Build history of the part. All positions in model axes, mm. Face numbers are marked on the shaded views. A direction names the side the tool comes from. Give positions to 0.01 mm unless a question says otherwise; leave off trailing zeros. Order: outer loops, then holes, each group sorted by start corner. A loop starts at its lowest first (then second) coordinate and runs counter-clockwise, first axis right, second up. Notation, with made-up numbers: M 81.25,16 L 85.25,16 A27 ccw 85.25,45 Z; hole C 53.5,59 d7. An arc over 180 degrees is marked long. One line per item, written item: value.
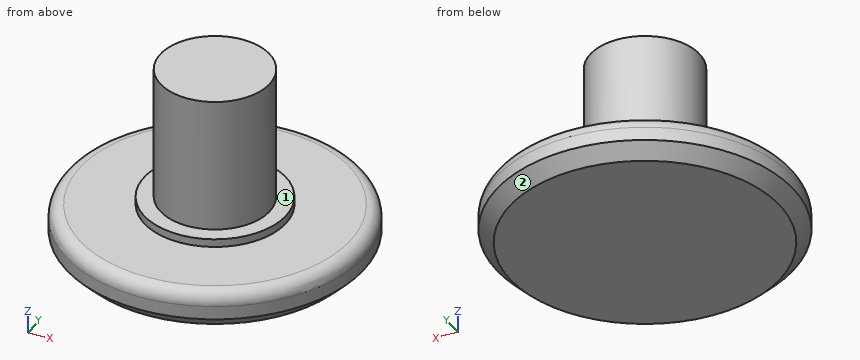
from build123d import *

# Parameters (mm, degrees)
F0_R     = 11
F1_DEPTH = 3
F2_R     = 5.25
F3_DEPTH = 0.6
F4_R     = 4.05
F5_DEPTH = 10
F6_SIZE  = 1
F7_R     = 1


with BuildPart() as f1:
    # F0 (on Top) → F1 (new body)
    with BuildSketch(Plane.XY):
        Circle(F0_R)
    extrude(amount=F1_DEPTH)

    # F2 (on face) → F3 (join)
    with BuildSketch(Plane.XY.offset(3)):
        Circle(F2_R)
    extrude(amount=F3_DEPTH)

    # F4 (on face) → F5 (join)
    with BuildSketch(Plane.XY.offset(3.6)):
        Circle(F4_R)
    extrude(amount=F5_DEPTH)

    # F6
    f6_edges = [f1.edges().sort_by_distance(p)[0] for p in [
        (-11, 0, 0),
    ]]
    chamfer(f6_edges, length=F6_SIZE)

    # F7
    f7_edges = [f1.edges().sort_by_distance(p)[0] for p in [
        (-11, 0, 3),
    ]]
    fillet(f7_edges, radius=F7_R)


solid = f1.part
1) Saw through at A-A, the plane y = 0. Write the cut outline in (x, z).
Check values:
outline: M -11,1 L -10,0 L 10,0 L 11,1 L 11,2 A1 ccw 10,3 L 5.25,3 L 5.25,3.6 L 4.05,3.6 L 4.05,13.6 L -4.05,13.6 L -4.05,3.6 L -5.25,3.6 L -5.25,3 L -10,3 A1 ccw -11,2 Z
2) Tool access for the marked faces 1 and 2: list every direction of +Z, -Z, +X, -X, +Y, -Y with a clear straight run to the whole face (end or side of a thin tool).
Check values:
face 1: +Z
face 2: -Z
3) Pin check, flat tips, straight feed: pin 1 (1.5 mm diameter, centred on x = 4.5, z = 2.5, fed in from -Y); pin 2 (4 mm diameter, centred on y = -6, z = 3, fed in from +X); pin 3 (3 mm diameter, centred on x = -1.5, z = 5, fed in from +Y). Stop position of each tip, or through.
Check values:
pin 1: y = -10.3
pin 2: x = 10.16
pin 3: y = 5.16
4) Drill centre lines: probe 1 along Z at (x, y) = (1.5, -4); probe 2 along Z at (x, y) = (-3.25, 7); probe 3 along Y at (x, z) = (2.5, 9.5). Where is each one in solid material? Low to high. Write a range as from..to.
Check values:
probe 1: 0..3.6
probe 2: 0..3
probe 3: -3.19..3.19
5) Saw through at C-C, the plane z = 12.25. Write the cut outline in (x, y).
Check values:
outline: C 0,0 d8.1
